The listing builds one solid part. Answer for the finished solid, in the listing's coordinates (mm). Face numbers are marked on the shaded views. A direction names the side the tool comes from. Round coordinates to 2 decimals unless told otherwise and drop trailing zeros. Order: outer loops, then holes, each group sorted by start corner. A loop starts at its lowest first (then second) coordinate and runs counter-clockwise, first axis right, second up. Notation, with made-up numbers: (24, 13.25) - (44, 13.25) arc R28 ccw to (44, 36.25) - close; hole circle Ø10 at (61, 40.25). An arc over 180 degrees is marked (long way). One line per item, written item: value. Start each with the question number.
1. Flat-ended cylindrical pins translate along their axes: P1, Ø12, axis at x = 15, y = 17.5, coming from the +Z side; P2, Ø4, axis at x = 9.5, z = -6.5, coming from the +Y side; P3, Ø1.5, axis at y = 15.5, z = -7, coming from the +X side. Find the tip coordinate at first contact, or state that the pin passes through.
2. Straight lines are drawn through the part: line 1 (X direction, y = 2.1, z = -11.25); line 2 (Z direction, x = 11, y = 19.5); line 3 (X direction, y = 15.5, z = 6). For each, find the intervals that lie inside material, in ascending order.
3. For a pull along Z with two mould halves and no side action, classify the marked faces 1, 2 and 3 as released by +Z, released by -Z, zero draft, split by the parting line, or undercut.
4. A tool of negligible diameter and unlimited length cuts with its end or side. For the marked faces 4, 5 and 6, from which of +Z, -Z, +X, -X, +Y, -Y can it reach the whole face along a straight path? Write none if from no direction.
5. Section C-C, the plane z = 22.5 is taken. Give the vertices of the cut face in (x, y), then the cut area to 3 significant figures.
6. Section B-B, the plane y = 4 is taken. Give the vertices of the cut face in (x, z) (3 decimals).
7. Section A-A, the plane z = -22 is taken. Give the vertices of the cut face in (x, y).
from build123d import *

# Parameters (mm, degrees)
ESBO_O1_R                = 28
RESSALTO_EXTRUS_O1_DEPTH = 5
ESBO_O6_R                = 10.75
CORTE_EXTRUS_O1_DEPTH    = 5
ESBO_O7_R                = 9
CORTE_EXTRUS_O2_DEPTH    = 0.4
CORTE_EXTRUS_O3_REACH    = 51.558
ESBO_O8_R                = 3.05
PADR_OCIRCULAR1_COUNT    = 3
CORTE_EXTRUS_O4_REACH    = 51.558
ESBO_O9_R                = 1.4
PADR_OCIRCULAR2_COUNT    = 3
PADR_OCIRCULAR3_COUNT    = 3
CHANFRO1_SIZE            = 2
CHANFRO2_SIZE            = 2
RESSALTO_EXTRUS_O2_DEPTH = 10.4
PADR_OCIRCULAR4_COUNT    = 15


with BuildPart() as part:
    # Esboço1 → Ressalto-extrusão1 (new body)
    with BuildSketch(Plane(origin=(0, 0, 0), x_dir=(1, 0, 0), z_dir=(0, 1, 0))):
        with Locations(Location((0, 0, 0), (0, 0, 270))):
            Circle(ESBO_O1_R)
    extrude(amount=RESSALTO_EXTRUS_O1_DEPTH)

    # Esboço5 → Revolução1 (revolve)
    with BuildSketch(Plane(origin=(0, 0, 0), x_dir=(0, 0, -1), z_dir=(1, 0, 0))):
        Polygon((0, 5), (-16.5, 5), (-14.5, 7), (-14.5, 9), (-12.3, 9), (-12.3, 12.4), (-9.37, 12.4), (-9.37, 22.8), (-7.5, 22.8), (-7.5, 23.8), (-5.5, 23.8), (-5.5, 29.8), (0, 29.8), align=None)
    revolve(axis=Axis((0, 29.8, 0), (0, -1, 0)))

    # Esboço6 → Corte-extrusão1 (cut)
    with BuildSketch(Plane.XZ):
        with Locations(Location((0, 0, 0), (0, 0, 270))):
            Circle(ESBO_O6_R)
    extrude(amount=-CORTE_EXTRUS_O1_DEPTH, mode=Mode.SUBTRACT)

    # Esboço7 → Corte-extrusão2 (cut)
    with BuildSketch(Plane.XZ.offset(-5)):
        with Locations(Location((0, 0, 0), (0, 0, 270))):
            Circle(ESBO_O7_R)
    extrude(amount=-CORTE_EXTRUS_O2_DEPTH, mode=Mode.SUBTRACT)

    # Esboço8 → Corte-extrusão3 (cut, up to next)
    with BuildSketch(Plane.XZ, mode=Mode.PRIVATE) as corte_extrus_o3_sk1:
        with Locations(Location((0, 22.5, 0), (0, 0, 270))):
            Circle(ESBO_O8_R)
    corte_extrus_o3_tool1 = extrude(corte_extrus_o3_sk1.sketch, amount=-CORTE_EXTRUS_O3_REACH, mode=Mode.PRIVATE) & part.part
    corte_extrus_o3 = corte_extrus_o3_tool1.solids().sort_by_distance((0, 0, 22.5))[0]
    add(corte_extrus_o3, mode=Mode.SUBTRACT)

    # PadrãoCircular1: Corte-extrusão3 ×3 about axis
    padr_ocircular1_axis = Axis((0, 0, 0), (0, 1, 0))
    for i in range(1, PADR_OCIRCULAR1_COUNT):
        add(corte_extrus_o3.rotate(padr_ocircular1_axis, i * 360 / PADR_OCIRCULAR1_COUNT), mode=Mode.SUBTRACT)

    # Esboço9 → Corte-extrusão4 (cut, up to next)
    with BuildSketch(Plane.XZ, mode=Mode.PRIVATE) as corte_extrus_o4_sk1:
        with Locations(Location((-19.052558883, 11, 0), (0, 0, 270))):
            Circle(ESBO_O9_R)
    corte_extrus_o4_tool1 = extrude(corte_extrus_o4_sk1.sketch, amount=-CORTE_EXTRUS_O4_REACH, mode=Mode.PRIVATE) & part.part
    corte_extrus_o4 = corte_extrus_o4_tool1.solids().sort_by_distance((-19.052559, 0, 11))[0]
    add(corte_extrus_o4, mode=Mode.SUBTRACT)

    # PadrãoCircular2: Corte-extrusão4 ×3 about axis
    padr_ocircular2_axis = Axis((0, 0, 0), (0, 1, 0))
    for i in range(1, PADR_OCIRCULAR2_COUNT):
        add(corte_extrus_o4.rotate(padr_ocircular2_axis, i * 360 / PADR_OCIRCULAR2_COUNT), mode=Mode.SUBTRACT)

    # Loft de corte1: read off the stored shape, not the designer's step
    # Loft de corte1: loft between two sections, ruled curve by curve
    loft_de_corte1_from = [
        Edge.make_bspline([(-18.260331243, 3, 17.20543513), (-17.315862444, 3, 16.040111704), (-16.150539018, 3, 16.984580503), (-17.095007817, 3, 18.149903929), (-18.039476615, 3, 19.315227355), (-19.204800042, 3, 18.370758556), (-18.260331243, 3, 17.20543513)], [0, 0, 0, 0, 0.5, 0.5, 0.5, 1, 1, 1, 1], 3, [1, 0.333333333, 0.333333333, 1, 0.333333333, 0.333333333, 1]),
    ]
    loft_de_corte1_to = [
        Edge.make_bspline([(-18.914864913, 0, 17.499210616), (-18.557947085, 0, 15.024819849), (-16.083556319, 0, 15.381737677), (-16.440474147, 0, 17.856128444), (-16.797391974, 0, 20.33051921), (-19.271782741, 0, 19.973601382), (-18.914864913, 0, 17.499210616)], [0, 0, 0, 0, 0.5, 0.5, 0.5, 1, 1, 1, 1], 3, [1, 0.333333333, 0.333333333, 1, 0.333333333, 0.333333333, 1]),
    ]
    loft_de_corte1 = Solid(Shell([*[Face.make_surface_from_curves(loft_de_corte1_from[k], loft_de_corte1_to[k]) for k in range(1)], Face(Wire(loft_de_corte1_from)), Face(Wire(loft_de_corte1_to))]))
    add(loft_de_corte1, mode=Mode.SUBTRACT)

    # PadrãoCircular3: Loft de corte1 ×3 about axis
    padr_ocircular3_axis = Axis((0, 0, 0), (0, 1, 0))
    for i in range(1, PADR_OCIRCULAR3_COUNT):
        add(loft_de_corte1.rotate(padr_ocircular3_axis, i * 360 / PADR_OCIRCULAR3_COUNT), mode=Mode.SUBTRACT)

    # Chanfro1
    chanfro1_edges = [part.edges().sort_by_distance(p)[0] for p in [
        (-19.052558883, 5, 12.4),
    ]]
    chamfer(chanfro1_edges, length=CHANFRO1_SIZE)

    # Chanfro2
    chanfro2_edges = [part.edges().sort_by_distance(p)[0] for p in [
        (20.264994449, 5, 10.3),
        (-1.212435565, 5, -22.7),
    ]]
    chamfer(chanfro2_edges, length=CHANFRO2_SIZE)

    # Esboço15 → Ressalto-extrusão2 (add)
    with BuildSketch(Plane(origin=(0, 22.8, 0), x_dir=(1, 0, 0), z_dir=(0, 1, 0))):
        with BuildLine():
            Line((0.335, 12.75), (-0.335, 12.75))
            ThreePointArc((-0.335, 12.75), (-1.106422887, 11.109098221), (-1.167760303, 9.296947664))
            ThreePointArc((-1.167760303, 9.296947664), (0, 9.37), (1.167760303, 9.296947664))
            ThreePointArc((1.167760303, 9.296947664), (1.106422887, 11.109098221), (0.335, 12.75))
        make_face()
    ressalto_extrus_o2 = extrude(amount=-RESSALTO_EXTRUS_O2_DEPTH)

    # PadrãoCircular4: Ressalto-extrusão2 ×15 about axis
    padr_ocircular4_axis = Axis((0, 0, 0), (0, 1, 0))
    for i in range(1, PADR_OCIRCULAR4_COUNT):
        add(ressalto_extrus_o2.rotate(padr_ocircular4_axis, i * 360 / PADR_OCIRCULAR4_COUNT))


solid = part.part
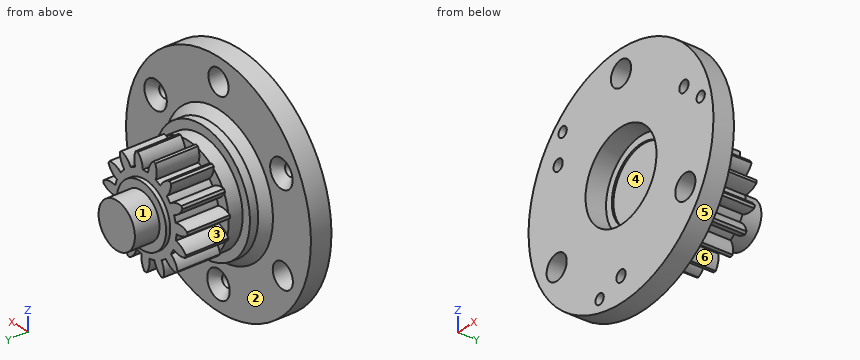
Answer list:
1. P1: stops at z = 6.7
1. P2: stops at y = 22.8
1. P3: stops at x = 9.56
2. line 1: x = -25.64 to -22.54, -16.44 to 16.44, 22.54 to 25.64
2. line 2: z = -4.48 to -2.44, 0.01 to 2.25, 5.66 to 6.45
2. line 3: x = -11.17 to -7.94, -7.2 to 7.2, 7.94 to 11.17
3. face 1: split by the parting line
3. face 2: zero draft
3. face 3: undercut
4. face 4: -Y
4. face 5: +Y, -Y
4. face 6: +Y
5. outline: (-16.67, 0) - (-3.05, 0) - (-3.05, 5) - (-16.67, 5) - close; (3.05, 0) - (16.67, 0) - (16.67, 5) - (3.05, 5) - close
5. area: 136 mm²
6. outline: circle Ø56 at (0, 0); hole circle Ø6.1 at (-19.486, -11.25); hole circle Ø4.8 at (-19.053, 11); hole circle Ø21.5 at (0, 0); hole circle Ø6.1 at (0, 22.5); hole circle Ø4.8 at (0, -22); hole circle Ø6.1 at (19.486, -11.25); hole circle Ø4.8 at (19.053, 11)
7. outline: (-17.32, 0) - (-1.4, 0) - (-1.4, 3) - (-3.4, 5) - (-17.32, 5) - close; (1.4, 0) - (17.32, 0) - (17.32, 5) - (3.4, 5) - (1.4, 3) - close
